Work out the finished part from the listing and answer in its coordinate system (mm). A direction names the side the tool comes from. Round coordinates to 2 decimals unless told otherwise and drop trailing zeros. Loops run counter-clockwise (first coordinate to the right, second up) from the corner with the lowest first, then second, coordinate; pieces in that order, holes last.
```python
from build123d import *

# Parameters (mm, degrees)
SKETCH1_R           = 0.75
BOSS_EXTRUDE1_DEPTH = 2.35
SKETCH2_R           = 1.5
CUT_EXTRUDE1_DEPTH  = 2.35
SKETCH3_R           = 4.18
SKETCH3_R_2         = 2.875
BOSS_EXTRUDE2_DEPTH = 2.75


with BuildPart() as part:
    # Sketch1 → Boss-Extrude1 (new body)
    with BuildSketch(Plane(origin=(0, 0, 0), x_dir=(1, 0, 0), z_dir=(0, 1, 0))):
        with BuildLine():
            Line((3.95, 6.84160069), (10.691342951, 8.482050808))
            ThreePointArc((10.691342951, 8.482050808), (13.423393759, 7.75), (12.691342951, 5.017949192))
            Line((12.691342951, 5.017949192), (7.9, 0))
            Line((7.9, 0), (12.691342951, -5.017949192))
            ThreePointArc((12.691342951, -5.017949192), (13.423393759, -7.75), (10.691342951, -8.482050808))
            Line((10.691342951, -8.482050808), (3.95, -6.84160069))
            Line((3.95, -6.84160069), (2, -13.5))
            ThreePointArc((2, -13.5), (0, -15.5), (-2, -13.5))
            Line((-2, -13.5), (-3.95, -6.84160069))
            Line((-3.95, -6.84160069), (-10.691342951, -8.482050808))
            ThreePointArc((-10.691342951, -8.482050808), (-13.423393759, -7.75), (-12.691342951, -5.017949192))
            Line((-12.691342951, -5.017949192), (-7.9, 0))
            Line((-7.9, 0), (-12.691342951, 5.017949192))
            ThreePointArc((-12.691342951, 5.017949192), (-13.423393759, 7.75), (-10.691342951, 8.482050808))
            Line((-10.691342951, 8.482050808), (-3.95, 6.84160069))
            Line((-3.95, 6.84160069), (-2, 13.5))
            ThreePointArc((-2, 13.5), (0, 15.5), (2, 13.5))
            Line((2, 13.5), (3.95, 6.84160069))
        make_face()
        with Locations((0, 10.5)):
            Circle(SKETCH1_R, mode=Mode.SUBTRACT)
        with Locations((0, 13.5)):
            Circle(SKETCH1_R, mode=Mode.SUBTRACT)
        with Locations((0, 7.5)):
            Circle(SKETCH1_R, mode=Mode.SUBTRACT)
        with Locations((11.691342951, 6.75)):
            Circle(SKETCH1_R, mode=Mode.SUBTRACT)
        with Locations((9.09326674, 5.25)):
            Circle(SKETCH1_R, mode=Mode.SUBTRACT)
        with Locations((6.495190528, 3.75)):
            Circle(SKETCH1_R, mode=Mode.SUBTRACT)
        with Locations((11.691342951, -6.75)):
            Circle(SKETCH1_R, mode=Mode.SUBTRACT)
        with Locations((9.09326674, -5.25)):
            Circle(SKETCH1_R, mode=Mode.SUBTRACT)
        with Locations((6.495190528, -3.75)):
            Circle(SKETCH1_R, mode=Mode.SUBTRACT)
        with Locations((0, -13.5)):
            Circle(SKETCH1_R, mode=Mode.SUBTRACT)
        with Locations((0, -10.5)):
            Circle(SKETCH1_R, mode=Mode.SUBTRACT)
        with Locations((0, -7.5)):
            Circle(SKETCH1_R, mode=Mode.SUBTRACT)
        with Locations((-11.691342951, -6.75)):
            Circle(SKETCH1_R, mode=Mode.SUBTRACT)
        with Locations((-9.09326674, -5.25)):
            Circle(SKETCH1_R, mode=Mode.SUBTRACT)
        with Locations((-6.495190528, -3.75)):
            Circle(SKETCH1_R, mode=Mode.SUBTRACT)
        with Locations((-11.691342951, 6.75)):
            Circle(SKETCH1_R, mode=Mode.SUBTRACT)
        with Locations((-9.09326674, 5.25)):
            Circle(SKETCH1_R, mode=Mode.SUBTRACT)
        with Locations((-6.495190528, 3.75)):
            Circle(SKETCH1_R, mode=Mode.SUBTRACT)
    extrude(amount=BOSS_EXTRUDE1_DEPTH)

    # Sketch2 → Cut-Extrude1 (cut)
    with BuildSketch(Plane(origin=(0, 2.35, 0), x_dir=(1, 0, 0), z_dir=(0, 1, 0))):
        Circle(SKETCH2_R)
    extrude(amount=-CUT_EXTRUDE1_DEPTH, mode=Mode.SUBTRACT)

    # Sketch3 → Boss-Extrude2 (add)
    with BuildSketch(Plane(origin=(0, 2.35, 0), x_dir=(1, 0, 0), z_dir=(0, 1, 0))):
        Circle(SKETCH3_R)
        Circle(SKETCH3_R_2, mode=Mode.SUBTRACT)
    extrude(amount=BOSS_EXTRUDE2_DEPTH)


solid = part.part
```
1. Given pin 1 (2.5 mm diameter, centred on x = 0, z = -13.5, fed in from +Y), flat-ended and moving along its own axis, determine where the tip first touches the part or whether it passes through.
Answer key:
pin 1: stops at y = 2.35
2. Find section D-D (x = -3.5). Write down the section's boundary in (y, z), then the cut area to 3 significant figures.
Answer key:
outline: (0, -8.38) - (2.35, -8.38) - (2.35, -2.29) - (5.1, -2.29) - (5.1, 2.29) - (2.35, 2.29) - (2.35, 8.38) - (0, 8.38) - close
area: 51.9 mm2
3. Determine the mould class of faces 5 (the face through (10.26, 1.16, 2.47)), 6 (the face through (2.96, 1.16, -10.22)), 7 (the face through (-10.329, 1.159, 2.544)), 8 (the face through (2.99, 1.16, 10.12)) for opening direction X: +X half, -X half, draft (parallel to the pull), parting line (faces both ways), or undercut.
Answer key:
face 5: +X half
face 6: undercut
face 7: -X half
face 8: undercut
4. Find section A-A (z = 0.5). Write down the section's boundary in (x, y).
Answer key:
outline: (-8.38, 0) - (-1.41, 0) - (-1.41, 2.35) - (-2.83, 2.35) - (-2.83, 5.1) - (-4.15, 5.1) - (-4.15, 2.35) - (-8.38, 2.35) - close; (1.41, 0) - (8.38, 0) - (8.38, 2.35) - (4.15, 2.35) - (4.15, 5.1) - (2.83, 5.1) - (2.83, 2.35) - (1.41, 2.35) - close
5. Find section C-C (y = 4.7). Write down the section's boundary in (x, z) (3 decimals).
Answer key:
outline: circle Ø8.36 at (0, 0); hole circle Ø5.75 at (0, 0)
6. Find section B-B (x = 11.5). Write down the section's boundary in (y, z).
Answer key:
outline: (0, -8.74) - (2.35, -8.74) - (2.35, -7.48) - (0, -7.48) - close; (0, -6.02) - (2.35, -6.02) - (2.35, -3.77) - (0, -3.77) - close; (0, 3.77) - (2.35, 3.77) - (2.35, 6.02) - (0, 6.02) - close; (0, 7.48) - (2.35, 7.48) - (2.35, 8.74) - (0, 8.74) - close
7. Which of the six approach directions +Z, -Z, +X, -X, +Y, -Y give full straight-line access (tool end or side, diameter ignored) to faces 1 (the face through (-7.27, 1.16, 7.65)), 2 (the face through (9.8, 1.2, -5.5)), 3 (the face through (7.27, 1.16, -7.65)), 4 (the face through (-1.2, 2.35, 1.2))?
Answer key:
face 1: +Z, +Y, -Y
face 2: +Y, -Y
face 3: -Z, +Y, -Y
face 4: +Y
8. Consider probe 1 along X at (y, z) = (1.6, 4); probe 2 along X at (y, z) = (1.6, 3.75); probe 3 along X at (y, z) = (3.45, 0) (3 decimals). Determine where each line is inside the solid, lowest interval first.
Answer key:
probe 1: x = -11.72 to -7.2, -5.79 to 5.79, 7.2 to 11.72
probe 2: x = -11.48 to -7.25, -5.75 to 5.75, 7.25 to 11.48
probe 3: x = -4.18 to -2.875, 2.875 to 4.18
